Could you check a few things on this model? Use its own coordinates, in mm. A direction names the side the tool comes from. Give positions to 0.01 mm unless a question says otherwise; leave off trailing zeros. Order: outer loops, then holes, each group sorted by start corner. A loop starts at its lowest first (then second) coordinate and runs counter-clockwise, first axis right, second up. Notation, with made-up numbers: (20, 85.25) -> (61, 85.25) arc R7 cw to (61, 90.25) -> close; hole circle Ø10 at (-11.75, 2.5). An arc over 180 degrees is marked (long way). Write each question's results on one line, items separated by ' | '.
```python
from build123d import *

# Parameters (mm, degrees)
SKETCH1_W               = 31
SKETCH1_H               = 36
SKETCH1_W_2             = 27
SKETCH1_H_2             = 32
EXTRUDE1_DEPTH          = 16.5
SKETCH2_W               = 32
SKETCH2_H               = 6
CUT_EXTRUDE1_DEPTH      = 40.462007045
CUT_EXTRUDE2_DEPTH      = 43.52646235
FILLET1_R               = 1
CUT_EXTRUDE4_DEPTH      = 43.52646235
CUT_EXTRUDE4_DEPTH_BACK = 43.52646235


with BuildPart() as part:
    # Sketch1 → Extrude1 (new body)
    with BuildSketch(Plane(origin=(0, 0, 0), x_dir=(1, 0, 0), z_dir=(0, 1, 0))):
        Rectangle(SKETCH1_W, SKETCH1_H)
        Rectangle(SKETCH1_W_2, SKETCH1_H_2, mode=Mode.SUBTRACT)
    extrude(amount=EXTRUDE1_DEPTH)

    # Sketch2 → Cut-Extrude1 (cut, through all)
    with BuildSketch(Plane.ZY.offset(15.5)):
        with Locations((0, 3)):
            Rectangle(SKETCH2_W, SKETCH2_H)
    extrude(amount=-CUT_EXTRUDE1_DEPTH, mode=Mode.SUBTRACT)

    # Sketch3 → Cut-Extrude2 (cut, through all)
    with BuildSketch(Plane(origin=(0, 0, -18), x_dir=(-1, 0, 0), z_dir=(0, 0, -1))):
        Polygon((-3.520725942, 16.5), (3.520725942, 16.5), (1.5, 13), (-1.5, 13), align=None)
    extrude(amount=-CUT_EXTRUDE2_DEPTH, mode=Mode.SUBTRACT)

    # Fillet1
    fillet1_edges = [part.edges().sort_by_distance(p)[0] for p in [
        (15.5, 16.5, 0),
        (-15.5, 16.5, 0),
    ]]
    fillet(fillet1_edges, radius=FILLET1_R)

    # Sketch4 → Cut-Extrude4 (cut, two sides: drawn at the far end of the back side and taken through both)
    with BuildSketch(Plane(origin=(0, 0, -18), x_dir=(-1, 0, 0), z_dir=(0, 0, -1)).offset(-CUT_EXTRUDE4_DEPTH_BACK)):
        with BuildLine():
            Line((-56.695317872, -48.043906057), (-8.415960011, 0))
            ThreePointArc((-8.415960011, 0), (0, 3.47396015), (8.415960011, 0))
            Line((8.415960011, 0), (56.695317872, -48.043906057))
            Line((56.695317872, -48.043906057), (56.695317872, -184.265979228))
            Line((56.695317872, -184.265979228), (-56.695317872, -184.265979228))
            Line((-56.695317872, -184.265979228), (-56.695317872, -48.043906057))
        make_face()
    extrude(amount=CUT_EXTRUDE4_DEPTH + CUT_EXTRUDE4_DEPTH_BACK, mode=Mode.SUBTRACT)


solid = part.part
```
Q1. I need wall thicknesses on line 1 along Z through (x, y) = (13, 3); line 2 along X through (y, z) = (13, -10); line 3 along Y through (x, z) = (14, 13). Which ranges of each line are inside material? Lowest first, please.
Here are the results:
line 1: z = -18 to -16, 16 to 18 | line 2: x = -15.5 to -13.5, 13.5 to 15.5 | line 3: y = 6 to 16.5
Q2. Suppose I cut it at A-A on x = 13. Please give me the cut outline in (y, z), and give its area (3 significant figures).
Here are the results:
outline: (0, -18) -> (16.5, -18) -> (16.5, -16) -> (0, -16) -> close; (0, 16) -> (16.5, 16) -> (16.5, 18) -> (0, 18) -> close | area: 66.0 mm²
Q3. Suppose I cut it at D-D on y = 9.25. Please give me the cut outline in (x, z).
Here are the results:
outline: (-15.5, -18) -> (15.5, -18) -> (15.5, 18) -> (-15.5, 18) -> close; hole (-13.5, -16) -> (13.5, -16) -> (13.5, 16) -> (-13.5, 16) -> close
Q4. Suppose I cut it at C-C on z = 3. Please give me the cut outline in (x, y).
Here are the results:
outline: (-15.5, 6) -> (-13.5, 6) -> (-13.5, 16.5) -> (-14.5, 16.5) arc R1 ccw to (-15.5, 15.5) -> close; (13.5, 6) -> (15.5, 6) -> (15.5, 15.5) arc R1 ccw to (14.5, 16.5) -> (13.5, 16.5) -> close
Q5. Suppose I cut it at B-B on y = 5.5. Please give me the cut outline in (x, z).
Here are the results:
outline: (-15.5, -18) -> (15.5, -18) -> (15.5, -16) -> (-15.5, -16) -> close; (-15.5, 16) -> (15.5, 16) -> (15.5, 18) -> (-15.5, 18) -> close
Q6. Thinking about a two-plate mould opening in Z: for faces 1 (the flat face through (0, 8, -18)), 2 (the flat face through (0, 13, -17)), 3 (the flat face through (-15, 6, 0)), which applies, +Z half, -Z half, draft (parallel to the pull), parting line (faces both ways), or undercut?
Here are the results:
face 1: -Z half | face 2: draft | face 3: undercut
Q7. For faces 4 (the cylindrical face through (-15.215, 16.199, -0.252)), 5 (the flat face through (2.5, 14.73, 16.99)), 6 (the flat face through (-13.5, 11, 0)), which set-ups out of +Z, -Z, +X, -X, +Y, -Y let a thin tool reach every point of the face, with its end or its side?
Here are the results:
face 4: +Z, -Z, -X, +Y | face 5: +Z, -Z, +Y | face 6: +Y, -Y
Q8. I'm going to push flat-ended pins straight in: pin 1 Ø0.6 at (x, z) = (-0.5, 16.5) entering from +Y; pin 2 Ø1.6 at (x, z) = (14.5, -1) entering from -Y. Where does each tip first touch, or does it pass through?
Here are the results:
pin 1: stops at y = 13 | pin 2: stops at y = 6
